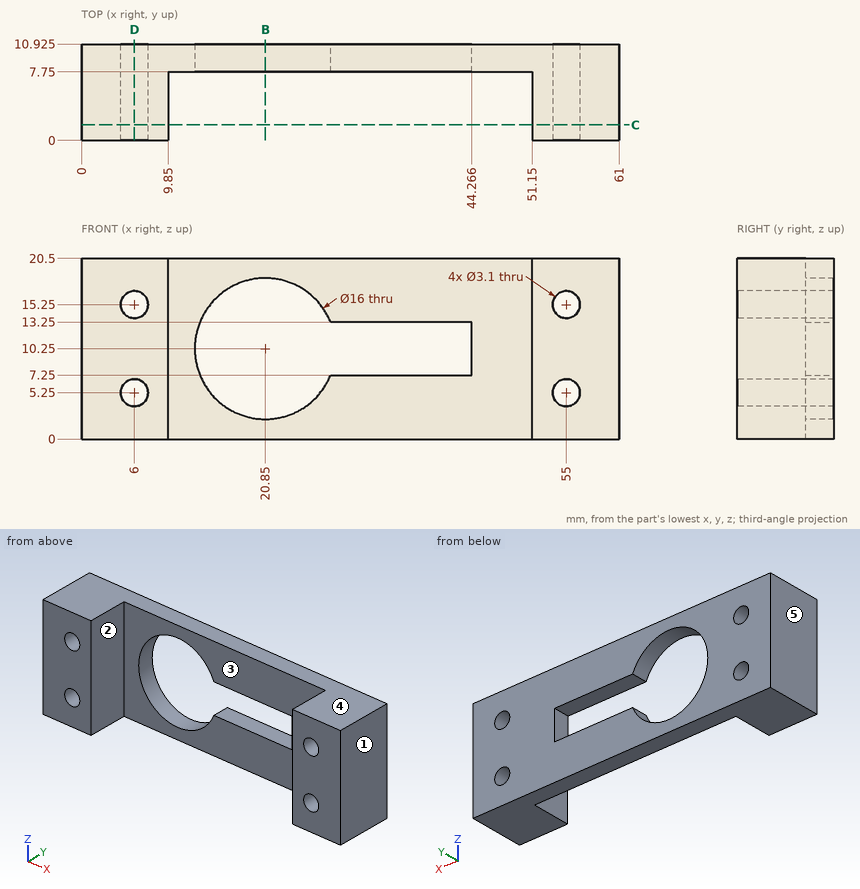
Geometry check sheet. Reference: drawing and pictorial views, mm from the part's lowest x, y, z. A direction names the side the tool comes from. Coordinates: 2 decimals unless noted, no trailing zeros. Write each loop counter-clockwise with the first axis right and the second up, starting at its lowest first coordinate (ties: lowest second). Pieces come first, ordered by that corner, then holes. Notation, with made-up numbers: (55.5, 57.25) - (79.5, 57.25) arc R19 cw to (79.5, 91.25) - close; hole circle Ø2 at (14.25, -13). An arc over 180 degrees is marked (long way). One line per question, with ' | ' between items. Start each with the question number.
1. Section check D-D (x = 6). Enter the section's corners in (y, z) (3 decimals).
2. Material ranges on line 1 along X through (y, z) = (7.5, 15.25); line 2 along Z through (x, y) = (55, 6.5); line 3 along Z through (x, y) = (20.85, 9.85), recorded low to high.
3. Section check B-B (x = 20.85). Enter the section's corners in (y, z) (3 decimals).
4. Access from +Z, -Z, +X, -X, +Y, -Y to the whole of each face (thin tool, end or side, straight path). Record for the marked faces 1 and 2.
5. Gauge pin test, flat ends, axial feed: P1, Ø12, axis at x = 27.5, z = 3, coming from the -Y side; P2, Ø1.9, axis at x = 6, z = 5.25, coming from the -Y side. Record the tip position at first contact, or that the pin passes through.
6. Draft check along X on the marked faces 3, 4 and 5. Enter one of: released by +X, released by -X, zero draft, split by the parting line, or undercut.
7. Section check C-C (y = 1.75). Enter the section's corners in (x, z).
Computed values:
1) outline: (0, 0) - (10.925, 0) - (10.925, 3.7) - (0, 3.7) - close; (0, 6.8) - (10.925, 6.8) - (10.925, 13.7) - (0, 13.7) - close; (0, 16.8) - (10.925, 16.8) - (10.925, 20.5) - (0, 20.5) - close
2) line 1: 0 to 4.45, 7.55 to 9.85, 51.15 to 53.45, 56.55 to 61 | line 2: 0 to 3.7, 6.8 to 13.7, 16.8 to 20.5 | line 3: 0 to 2.25, 18.25 to 20.5
3) outline: (7.75, 0) - (10.925, 0) - (10.925, 2.25) - (7.75, 2.25) - close; (7.75, 18.25) - (10.925, 18.25) - (10.925, 20.5) - (7.75, 20.5) - close
4) face 1: +Z, -Z, +X, +Y, -Y | face 2: +Z, -Z, -Y
5) P1: y = 7.75 | P2: through
6) face 3: undercut | face 4: zero draft | face 5: released by -X
7) outline: (0, 0) - (9.85, 0) - (9.85, 20.5) - (0, 20.5) - close; (51.15, 0) - (61, 0) - (61, 20.5) - (51.15, 20.5) - close; hole circle Ø3.1 at (6, 5.25); hole circle Ø3.1 at (6, 15.25); hole circle Ø3.1 at (55, 5.25); hole circle Ø3.1 at (55, 15.25)
